```python
from build123d import *

# Parameters (mm, degrees)
SKETCH_1_R          = 45
SKETCH_1_R_2        = 21
EXTRUDE_1_DEPTH     = 10
SKETCH_2_R          = 33
SKETCH_2_R_2        = 21
EXTRUDE_2_DEPTH     = 3
CUT_EXTRUDE_1_DEPTH = 88.964820488
SKETCH_5_R          = 26
CUT_EXTRUDE_2_DEPTH = 6


with BuildPart() as part:
    # 草图1 → 凸台-拉伸1 (new body)
    with BuildSketch(Plane.XY):
        with Locations((0, 29.456763584)):
            Circle(SKETCH_1_R)
        with Locations((0, 29.456763584)):
            Circle(SKETCH_1_R_2, mode=Mode.SUBTRACT)
    extrude(amount=EXTRUDE_1_DEPTH)

    # 草图2 → 凸台-拉伸2 (add)
    with BuildSketch(Plane.XY.offset(10)):
        with Locations((0, 29.456763584)):
            Circle(SKETCH_2_R)
        with Locations((0, 29.456763584)):
            Circle(SKETCH_2_R_2, mode=Mode.SUBTRACT)
    extrude(amount=EXTRUDE_2_DEPTH)

    # 草图4 → 切除-拉伸1 (cut, through all)
    with BuildSketch(Plane(origin=(0, 0, 0), x_dir=(-1, 0, 0), z_dir=(0, 0, -1))):
        with BuildLine():
            Line((-20.615528128, -10.543236416), (20.615528128, -10.543236416))
            ThreePointArc((20.615528128, -10.543236416), (0, -15.543236416), (-20.615528128, -10.543236416))
        make_face()
    extrude(amount=-CUT_EXTRUDE_1_DEPTH, mode=Mode.SUBTRACT)

    # 草图5 → 切除-拉伸2 (cut)
    with BuildSketch(Plane.XY.offset(13)):
        with Locations((0, 29.456763584)):
            Circle(SKETCH_5_R)
    extrude(amount=-CUT_EXTRUDE_2_DEPTH, mode=Mode.SUBTRACT)


solid = part.part
```
Model file for the job. Use its own axes, mm. A direction names the side the tool comes from. Coordinates: 2 decimals unless noted, no trailing zeros. Write each loop counter-clockwise with the first axis right and the second up, starting at its lowest first coordinate (ties: lowest second). Pieces come first, ordered by that corner, then holes. Notation, with made-up numbers: (-7, 67.25) - (40, 67.25) arc R32 cw to (40, 94.25) - close; hole circle Ø6 at (49.25, 75.25). An arc over 180 degrees is marked (long way). One line per question, with ' | ' between items. Start each with the question number.
Q1. 3-axis set-ups, long thin cutter, end or side, ignore diameter. For faces 4 (the face through (13, 60, 10)), 5 (the face through (1.679, 74.425, 4.93)): which of +Z, -Z, +X, -X, +Y, -Y reach the whole face in a straight line?
Q2. Drill centre lines: line 1 (Y direction, x = 0, z = 3.75); line 2 (Y direction, x = 0, z = 9.85); line 3 (X direction, y = 29, z = 4). Where is each one in solid material? Low to high. Write a range as [from, to].
Q3. Cut at C-C, the plane z = 2.5. List the corners of the cut face in (x, y), then the cut area to 3 significant figures.
Q4. Pin check, flat tips, straight feed: pin 1 (1 mm diameter, centred on y = -1.5, z = 4.5, fed in from -X); pin 2 (5 mm diameter, centred on x = 12, z = 7, fed in from +Y); pin 3 (1.5 mm diameter, centred on y = 31, z = 7.5, fed in from -X). Stop position of each tip, or through.
Q5. Cut at D-D, the plane x = -31. List the corners of the cut face in (y, z).
Q6. Cut at B-B, the plane y = 22. List the corners of the cut face in (x, z).
Q7. Cut at A-A, the plane x = 0. List the corners of the cut face in (y, z), then the cut area to 3 significant figures.
Q8. Pull direction X, two halves, no side cores. Call faces 1 (the face through (2, 51, 7)), 2 (the face through (-1, 51, 0)), 3 (the face through (-7.15, -2.76, 11.48)): pulls with the +X half, pulls with the -X half, needs draft (parallel to the pull), parting line crosses it, or undercut.
Answer below:
1) face 4: +Z | face 5: +Z, -Z
2) line 1: [-10.54, 8.46], [50.46, 74.46] | line 2: [-10.54, 3.46], [55.46, 74.46] | line 3: [-45, -21], [21, 45]
3) outline: (-20.62, -10.54) - (20.62, -10.54) arc R45 ccw (long way) to start; hole circle Ø42 at (0, 29.46) | area: 4,840 mm^2
4) pin 1: x = -33.13 | pin 2: y = 73.44 | pin 3: x = -44.99
5) outline: (-3.16, 0) - (62.08, 0) - (62.08, 10) - (40.77, 10) - (40.77, 13) - (18.14, 13) - (18.14, 10) - (-3.16, 10) - close
6) outline: (-44.38, 0) - (-19.63, 0) - (-19.63, 7) - (-24.91, 7) - (-24.91, 13) - (-32.15, 13) - (-32.15, 10) - (-44.38, 10) - close; (19.63, 0) - (44.38, 0) - (44.38, 10) - (32.15, 10) - (32.15, 13) - (24.91, 13) - (24.91, 7) - (19.63, 7) - close
7) outline: (-10.54, 0) - (8.46, 0) - (8.46, 7) - (3.46, 7) - (3.46, 13) - (-3.54, 13) - (-3.54, 10) - (-10.54, 10) - close; (50.46, 0) - (74.46, 0) - (74.46, 10) - (62.46, 10) - (62.46, 13) - (55.46, 13) - (55.46, 7) - (50.46, 7) - close | area: 442 mm^2
8) face 1: undercut | face 2: needs draft | face 3: parting line crosses it
